Geometry check sheet. Reference: drawing and pictorial views, mm from the part's lowest x, y, z. A direction names the side the tool comes from. Round coordinates to 2 decimals unless told otherwise and drop trailing zeros. Loops run counter-clockwise (first coordinate to the right, second up) from the corner with the lowest first, then second, coordinate; pieces in that order, holes last. Notation, with made-up numbers: (52, 86.25) -> (69, 86.25) arc R12 ccw to (69, 98.25) -> close; hole circle Ø3 at (22.5, 21.25). An arc over 180 degrees is marked (long way). Use one line per item in the form item = value. Start each with the question number.
(1) Material ranges on probe 1 along Y at (x, z) = (23, 4.5); probe 2 along Y at (x, z) = (42, 5); probe 3 along Z at (x, y) = (34.5, 13.25), recorded low to high. Write a range as [from, to].
(2) Sectioned sample at D-D (y = 21.25). Record the cut outline in (x, z).
(3) Sectioned sample at A-A (y = 12). Record the cut outline in (x, z).
(4) Go/stop test with flat-tipped pins: pin 1 (1.2 mm diameter, centred on x = 5.5, z = 8, fed in from -Y); pin 2 (1.9 mm diameter, centred on y = 9.5, z = 7.5, fed in from +X); pin 3 (4 mm diameter, centred on x = 41, y = 15, fed in from +Z); pin 4 (2 mm diameter, centred on y = 15, z = 4, fed in from -X). Record where each tip stops, or that it passes through.
(5) Draft check along Y on the marked faces 1, 2 and 3. Enter one of: released by +Y, released by -Y, zero draft, split by the parting line, or undercut.
(6) Sectioned sample at B-B (x = 23). Record the cut outline in (y, z).
(7) Sectioned sample at C-C (z = 8.25). Record the cut outline in (x, y), and give its area (3 significant figures).
(8) Set-up check for the marked faces 4, 5 and 6: record each of +Z, -Z, +X, -X, +Y, -Y from which the full face is reachable in a straight line by a thin tool's end or side.
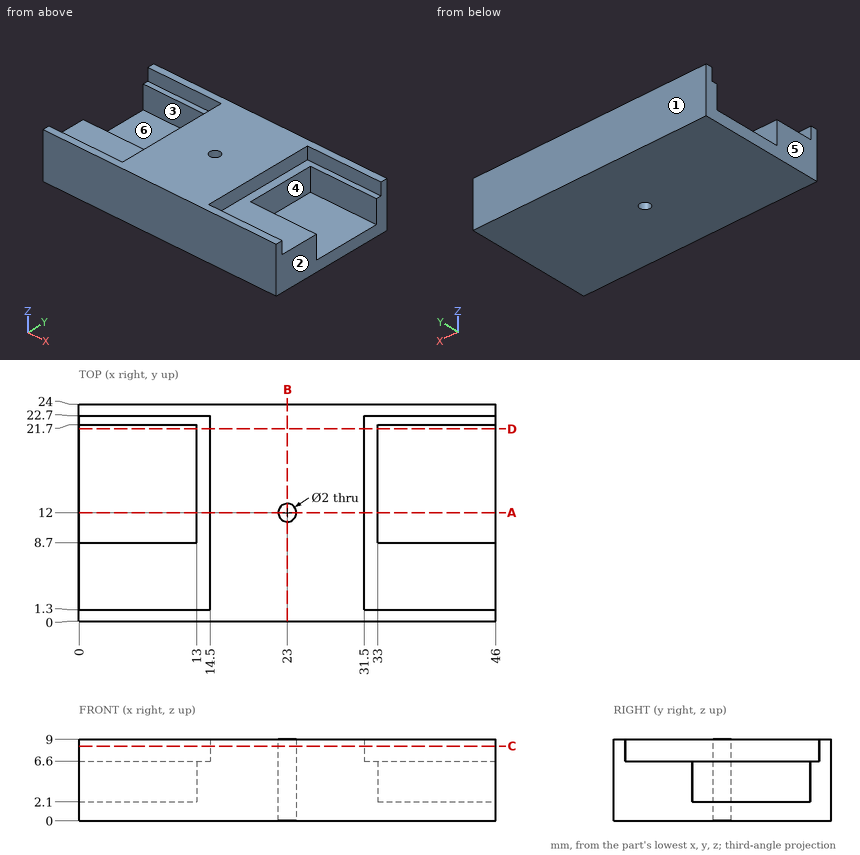
Checks:
q1.probe_1 = [0, 11], [13, 24]
q1.probe_2 = [0, 8.7], [21.7, 24]
q1.probe_3 = [0, 2.1]
q2.outline = (0, 0) -> (46, 0) -> (46, 2.1) -> (33, 2.1) -> (33, 6.6) -> (31.5, 6.6) -> (31.5, 9) -> (14.5, 9) -> (14.5, 6.6) -> (13, 6.6) -> (13, 2.1) -> (0, 2.1) -> close
q3.outline = (0, 0) -> (22, 0) -> (22, 9) -> (14.5, 9) -> (14.5, 6.6) -> (13, 6.6) -> (13, 2.1) -> (0, 2.1) -> close; (24, 0) -> (46, 0) -> (46, 2.1) -> (33, 2.1) -> (33, 6.6) -> (31.5, 6.6) -> (31.5, 9) -> (24, 9) -> close
q4.pin_1 = 0
q4.pin_2 = 33
q4.pin_3 = 2.1
q4.pin_4 = 13
q5.face_1 = released by +Y
q5.face_2 = zero draft
q5.face_3 = undercut
q6.outline = (0, 0) -> (11, 0) -> (11, 9) -> (0, 9) -> close; (13, 0) -> (24, 0) -> (24, 9) -> (13, 9) -> close
q7.outline = (0, 0) -> (46, 0) -> (46, 1.3) -> (31.5, 1.3) -> (31.5, 22.7) -> (46, 22.7) -> (46, 24) -> (0, 24) -> (0, 22.7) -> (14.5, 22.7) -> (14.5, 1.3) -> (0, 1.3) -> close; hole circle Ø2 at (23, 12)
q7.area = 480 mm2
q8.face_4 = +Z, +X
q8.face_5 = +Z, -Z, -X, +Y, -Y
q8.face_6 = +Z, -X
